Check sheet for the modelled part. Datum: model origin and axes. Units: mm. A direction names the side the tool comes from. Round coordinates to 2 decimals unless told otherwise and drop trailing zeros. Write each loop counter-clockwise with the first axis right and the second up, starting at its lowest first coordinate (ties: lowest second). Pieces come first, ordered by that corner, then holes. Notation, with made-up numbers: M -20.5,0 L -9.5,0 A19 cw -9.5,28 Z; hole C -8.5,39.5 d2. An arc over 180 degrees is marked long. One line per item, written item: value.
from build123d import *

# Parameters (mm, degrees)
BOSS_EXTRUDE1_DEPTH              = 6.35
F_21_64_0_32813_DIAMETER_HOLE1_D = 8.334502
LPATTERN1_COUNT                  = 2
LPATTERN1_PITCH                  = 38.1
LPATTERN1_COUNT_DIR2             = 2
LPATTERN1_PITCH_DIR2             = 38.1
F_21_64_0_32813_DIAMETER_HOLE2_D = 8.334502
LPATTERN2_COUNT                  = 3
LPATTERN2_PITCH                  = 50.8
LPATTERN2_COUNT_DIR2             = 2
LPATTERN2_PITCH_DIR2             = 38.1
SKETCH7_W                        = 9.525
SKETCH7_H                        = 88.9
CUT_EXTRUDE1_DEPTH               = 244.088107491
FILLET1_R                        = 6.35


with BuildPart() as part:
    # Sketch2 → Boss-Extrude1 (new body)
    with BuildSketch(Plane.XY):
        Polygon((0, 0), (76.2, 0), (76.2, 217.469814476), (58.378218394, 230.748923082), (0, 152.4), align=None)
    extrude(amount=BOSS_EXTRUDE1_DEPTH)

    # 21/64 (0.32813) Diameter Hole1 (through all)
    with Locations(Plane.XY.offset(6.35)):
        with Locations((57.15, 19.05)):
            f_21_64_0_32813_diameter_hole1 = Hole(F_21_64_0_32813_DIAMETER_HOLE1_D / 2)

    # LPattern1: 21_64 _0.32813_ Diameter Hole1 2 × 2
    with Locations(*[(-i * LPATTERN1_PITCH, j * LPATTERN1_PITCH_DIR2, 0) for i in range(LPATTERN1_COUNT) for j in range(LPATTERN1_COUNT_DIR2) if (i, j) != (0, 0)]):
        add(f_21_64_0_32813_diameter_hole1, mode=Mode.SUBTRACT)

    # 21/64 (0.32813) Diameter Hole2 (through all)
    with Locations(Plane.XY.offset(6.35)):
        with Locations((57.15, 197.2169065)):
            f_21_64_0_32813_diameter_hole2 = Hole(F_21_64_0_32813_DIAMETER_HOLE2_D / 2)

    # LPattern2: 21_64 _0.32813_ Diameter Hole2 3 × 2, 2 skipped
    with Locations(*[Vector(-0.597485201625335, -0.8018799372965586, 0) * (i * LPATTERN2_PITCH) + Vector(0.8018799372965592, -0.5974852016253344, 0) * (j * LPATTERN2_PITCH_DIR2) for i in range(LPATTERN2_COUNT) for j in range(LPATTERN2_COUNT_DIR2) if (i, j) not in ((0, 0), (0, 1), (2, 0))]):
        add(f_21_64_0_32813_diameter_hole2, mode=Mode.SUBTRACT)

    # Sketch7 → Cut-Extrude1 (cut, through all)
    with BuildSketch(Plane.XY.offset(6.35)):
        with Locations((71.4375, 44.45)):
            Rectangle(SKETCH7_W, SKETCH7_H)
    extrude(amount=-CUT_EXTRUDE1_DEPTH, mode=Mode.SUBTRACT)

    # Fillet1
    fillet1_edges = [part.edges().sort_by_distance(p)[0] for p in [
        (66.675, 88.9, 3.175),
    ]]
    fillet(fillet1_edges, radius=FILLET1_R)


solid = part.part
Q1. Sectioned sample at B-B on y = 19.05. Enter the section's corners in (x, z) (3 decimals), and give its area (3 significant figures).
Completed:
outline: M 0,0 L 14.883,0 L 14.883,6.35 L 0,6.35 Z; M 23.217,0 L 52.983,0 L 52.983,6.35 L 23.217,6.35 Z; M 61.317,0 L 66.675,0 L 66.675,6.35 L 61.317,6.35 Z
area: 318 mm^2
Q2. Sectioned sample at C-C on z = 2. State how many separate pieces and enclosed holes the cut face has, and give its area (3 significant figures).
Completed:
separate pieces: 1
enclosed holes: 8
area: 13,900 mm^2
Q3. Access from +Z, -Z, +X, -X, +Y, -Y to the whole of each face (thin tool, end or side, straight path). Record for faces 1 (the flat face through (66.675, 41, 3)), 2 (the flat face through (38, 117, 0)).
Completed:
face 1: +Z, -Z, +X, -Y
face 2: -Z, +X, -X, +Y, -Y
Q4. Draft check along Y on faces 3 (the cylindrical face through (24.557, 159.995, 3.131)), 4 (the flat face through (33, 0, 3)), 5 (the flat face through (76.2, 152, 3)). Enter one of: pulls with the +Y half, pulls with the -Y half, needs draft (parallel to the pull), parting line crosses it, or undercut.
Completed:
face 3: undercut
face 4: pulls with the -Y half
face 5: needs draft
Q5. Scan lines: line 1 (X direction, y = 93, z = 3.5); line 2 (Y direction, x = 19.05, z = 2.5); line 3 (Y direction, x = 16, z = 2). Record each from-to range of solid material in increasing order. Write a range as [from, to].
Completed:
line 1: [0, 22.83], [31.16, 76.2]
line 2: [0, 14.88], [23.22, 52.98], [61.32, 177.97]
line 3: [0, 16.21], [21.89, 54.31], [59.99, 173.87]
Q6. Sectioned sample at A-A on x = 26.5. Enter the section's corners in (y, z).
Completed:
outline: M 0,0 L 88.84,0 L 88.84,6.35 L 0,6.35 Z; M 97.12,0 L 152.32,0 L 152.32,6.35 L 97.12,6.35 Z; M 160.64,0 L 187.97,0 L 187.97,6.35 L 160.64,6.35 Z
Q7. Depth check by flat-ended pin: P1, Ø2.5, axis at x = 75, z = 2.5, coming from the -Y side. Enter the tip coordinate at first touch or a pass-through.
Completed:
P1: y = 88.9
Q8. Sectioned sample at D-D on y = 70. Enter the section's corners in (x, z) (3 decimals), and give its area (3 significant figures).
Completed:
outline: M 0,0 L 66.675,0 L 66.675,6.35 L 0,6.35 Z
area: 423 mm^2
